from build123d import *

# Parameters (mm, degrees)
SKETCH_1_W          = 32
SKETCH_1_H          = 22
EXTRUDE_1_DEPTH     = 3
SKETCH_2_W          = 3
SKETCH_2_H          = 22
EXTRUDE_2_DEPTH     = 8
SKETCH_3_R          = 1.5
CUT_EXTRUDE_1_DEPTH = 36.580893749
SKETCH_4_R          = 5.25
SKETCH_4_R_2        = 1.5
CUT_EXTRUDE_2_DEPTH = 22


with BuildPart() as part:
    # 草图1 → 凸台-拉伸1 (new body)
    with BuildSketch(Plane(origin=(0, 0, 0), x_dir=(1, 0, 0), z_dir=(0, 1, 0))):
        Rectangle(SKETCH_1_W, SKETCH_1_H)
    extrude(amount=EXTRUDE_1_DEPTH)

    # 草图2 → 凸台-拉伸2 (add)
    with BuildSketch(Plane(origin=(0, 3, 0), x_dir=(1, 0, 0), z_dir=(0, 1, 0))):
        with Locations((-14.5, 0)):
            Rectangle(SKETCH_2_W, SKETCH_2_H)
        with Locations((14.5, 0)):
            Rectangle(SKETCH_2_W, SKETCH_2_H)
    extrude(amount=EXTRUDE_2_DEPTH)

    # 草图3 → 切除-拉伸1 (cut, through all)
    with BuildSketch(Plane(origin=(16, 0, 0), x_dir=(0, 0, -1), z_dir=(1, 0, 0))):
        with Locations((-7, 7)):
            Circle(SKETCH_3_R)
        with Locations((7, 7)):
            Circle(SKETCH_3_R)
    extrude(amount=-CUT_EXTRUDE_1_DEPTH, mode=Mode.SUBTRACT)

    # 草图4 → 切除-拉伸2 (cut, through all)
    with BuildSketch(Plane(origin=(0, 3, 0), x_dir=(1, 0, 0), z_dir=(0, 1, 0))):
        with Locations(Location((0, 0, 0), (0, 0, 270))):
            Circle(SKETCH_4_R)
        with Locations(Location((0, 8, 0), (0, 0, 270))):
            Circle(SKETCH_4_R_2)
        with Locations(Location((8, 0, 0), (0, 0, 270))):
            Circle(SKETCH_4_R_2)
        with Locations(Location((0, -8, 0), (0, 0, 270))):
            Circle(SKETCH_4_R_2)
        with Locations(Location((-8, 0, 0), (0, 0, 270))):
            Circle(SKETCH_4_R_2)
    extrude(amount=-CUT_EXTRUDE_2_DEPTH, mode=Mode.SUBTRACT)


solid = part.part
Read the model definition and answer for the solid it produces. Units are mm, in the model's axes. A direction names the side the tool comes from. Round coordinates to 2 decimals unless told otherwise and drop trailing zeros. Write each loop counter-clockwise with the first axis right and the second up, starting at its lowest first coordinate (ties: lowest second). Pieces come first, ordered by that corner, then holes. Notation, with made-up numbers: M -27.75,7 L 11.25,7 A20 cw 11.25,27 Z; hole C -31,-39.75 d5. An arc over 180 degrees is marked long. Use a Markdown table: item, result.
1) The part is cut by section B-B (z = 0). Write down the section's boundary in (x, y).
Answers follow:
| item | result |
|---|---|
| outline | M -16,0 L -9.5,0 L -9.5,3 L -13,3 L -13,11 L -16,11 Z; M -6.5,0 L -5.25,0 L -5.25,3 L -6.5,3 Z; M 5.25,0 L 6.5,0 L 6.5,3 L 5.25,3 Z; M 9.5,0 L 16,0 L 16,11 L 13,11 L 13,3 L 9.5,3 Z |
2) The part is cut by section C-C (x = -8). Write down the section's boundary in (y, z), plus the area to 3 significant figures.
Answers follow:
| item | result |
|---|---|
| outline | M 0,-11 L 3,-11 L 3,-1.5 L 0,-1.5 Z; M 0,1.5 L 3,1.5 L 3,11 L 0,11 Z |
| area | 57.0 mm2 |
3) Flat-ended cylindrical pins translate along their axes: pin 1 (2.5 mm diameter, centred on x = 0, z = 8, fed in from +Y) (1 decimal); pin 2 (3.5 mm diameter, centred on y = 7, z = 7, fed in from -X); pin 3 (6 mm diameter, centred on x = 3.5, z = -8, fed in from +Y). Find the tip coordinate at first contact, or state that the pin passes through.
Answers follow:
| item | result |
|---|---|
| pin 1 | passes through |
| pin 2 | stops at x = -16 |
| pin 3 | stops at y = 3 |
4) Straight lines are drawn through the part: line 1 along X through (y, z) = (0.95, 0); line 2 along X through (y, z) = (6.75, -5.25); line 3 along X through (y, z) = (0.65, 8). For each, find the intervals that lie inside material, in ascending order. Write a range as [from, to].
Answers follow:
| item | result |
|---|---|
| line 1 | x = [-16, -9.5], [-6.5, -5.25], [5.25, 6.5], [9.5, 16] |
| line 2 | x = [-16, -13], [13, 16] |
| line 3 | x = [-16, -1.5], [1.5, 16] |
5) A tool of negligible diameter and unlimited length cuts with its end or side. For faces 4 (the flat face through (-3, 3, -5)), 5 (the cylindrical face through (6.536, 1.521, -0.325)), from which of +Z, -Z, +X, -X, +Y, -Y can it reach the whole face along a straight path? Write none if from no direction.
Answers follow:
| item | result |
|---|---|
| face 4 | +Z, -Z, +Y |
| face 5 | +Y, -Y |
6) The part is cut by section D-D (y = 9.75). Write down the section's boundary in (x, z), plus the area to 3 significant figures.
Answers follow:
| item | result |
|---|---|
| outline | M -16,-11 L -13,-11 L -13,11 L -16,11 Z; M 13,-11 L 16,-11 L 16,11 L 13,11 Z |
| area | 132 mm2 |
7) The part is cut by section A-A (y = 7). Write down the section's boundary in (x, z).
Answers follow:
| item | result |
|---|---|
| outline | M -16,-11 L -13,-11 L -13,-8.5 L -16,-8.5 Z; M -16,-5.5 L -13,-5.5 L -13,5.5 L -16,5.5 Z; M -16,8.5 L -13,8.5 L -13,11 L -16,11 Z; M 13,-11 L 16,-11 L 16,-8.5 L 13,-8.5 Z; M 13,-5.5 L 16,-5.5 L 16,5.5 L 13,5.5 Z; M 13,8.5 L 16,8.5 L 16,11 L 13,11 Z |
8) For a pull along X with two mould halves and no side action, classify faces 1 (the flat face through (16, 5, 0)), 2 (the cylindrical face through (1.6, 1.5, 5)), 3 (the flat face through (0, 2, 11)) as pulls with the +X half, pulls with the -X half, needs draft (parallel to the pull), parting line crosses it, or undercut.
Answers follow:
| item | result |
|---|---|
| face 1 | pulls with the +X half |
| face 2 | undercut |
| face 3 | needs draft |
